Geometry check sheet. Reference: the model listing, model coordinates, mm. A direction names the side the tool comes from. Round coordinates to 2 decimals unless told otherwise and drop trailing zeros. Order: outer loops, then holes, each group sorted by start corner. A loop starts at its lowest first (then second) coordinate and runs counter-clockwise, first axis right, second up. Notation, with made-up numbers: (24.5, 36.5) - (45.5, 36.5) arc R29 cw to (45.5, 59.5) - close; hole circle Ø3 at (84.25, -4.5). An arc over 180 degrees is marked (long way). Answer as CSV lines item,"result". Start each with the question number.
```python
from build123d import *

# Parameters (mm, degrees)
F0_W     = 100
F0_H     = 100
F1_DEPTH = 25
F3_DEPTH = 25


with BuildPart() as f1:
    # F0 (on Top) → F1 (new body)
    with BuildSketch(Plane.XY):
        Rectangle(F0_W, F0_H)
    extrude(amount=-F1_DEPTH)

    # F2 (on face) → F3 (join)
    with BuildSketch(Plane.XY):
        Polygon((16.568542, 40), (-16.568542, 40), (-40, 16.568542), (-40, -16.568542), (-16.568542, -40), (16.568542, -40), (40, -16.568542), (40, 16.568542), align=None)
    extrude(amount=F3_DEPTH)


solid = f1.part
```
1. Access from +Z, -Z, +X, -X, +Y, -Y to the whole of each face (thin tool, end or side, straight path). Record for faces 1 (the face through (0, -40, 12)), 2 (the face through (-23, 34, 0)), 3 (the face through (40, 0, 12)), 4 (the face through (0, 40, 12)), 5 (the face through (-28.12, 28.45, 12.32)).
2. Go/stop test with flat-tipped pins: pin 1 Ø12 at (y, z) = (-36, 12) entering from +X; pin 2 Ø20 at (x, z) = (-6, 11) entering from -Y; pin 3 Ø12.5 at (x, z) = (-5.5, 11) entering from +Y. Record where each tip stops, or that it passes through.
3. Thickness scan on probe 1 along Y at (x, z) = (-7.5, 15); probe 2 along Z at (x, y) = (-28.5, -39); probe 3 along Y at (x, z) = (25.5, 4.5). Record the ranges inside material, lowest first.
4. Section check A-A on x = 13. Record the boundary of the cut face in (y, z), plus the area to 3 significant figures.
5. Draft check along X on faces 6 (the face through (28.45, 28.12, 12.32)), 7 (the face through (-1, 50, -12)), 8 (the face through (-40, 0, 12)). Enter one of: released by +X, released by -X, zero draft, split by the parting line, or undercut.
Numbers:
1,face 1,"+Z, +X, -X, -Y"
1,face 2,"+Z"
1,face 3,"+Z, +X, +Y, -Y"
1,face 4,"+Z, +X, -X, +Y"
1,face 5,"+Z, -X, +Y"
2,pin 1,"stops at x = 26.57"
2,pin 2,"stops at y = -40"
2,pin 3,"stops at y = 40"
3,probe 1,"y = -40 to 40"
3,probe 2,"z = -25 to 0"
3,probe 3,"y = -31.07 to 31.07"
4,outline,"(-50, -25) - (50, -25) - (50, 0) - (40, 0) - (40, 25) - (-40, 25) - (-40, 0) - (-50, 0) - close"
4,area,"4,500 mm2"
5,face 6,"released by +X"
5,face 7,"zero draft"
5,face 8,"released by -X"
